Geometry: see drawing. Coordinates: mm, zero at the bounding-box minimum. A direction names the side the tool comes from. Give positions to 0.01 mm unless a question says otherwise; leave off trailing zeros. Write each loop counter-clockwise with the first axis right and the second up, starting at its lowest first coordinate (ties: lowest second). Pieces come first, ordered by that corner, then holes. Notation, with made-up numbers: M 64,38 L 95,38 A28 cw 95,67 Z; hole C 31,-34 d7. An arc over 180 degrees is marked long. Answer as a JSON object with one key per item and string values. Group by question number.
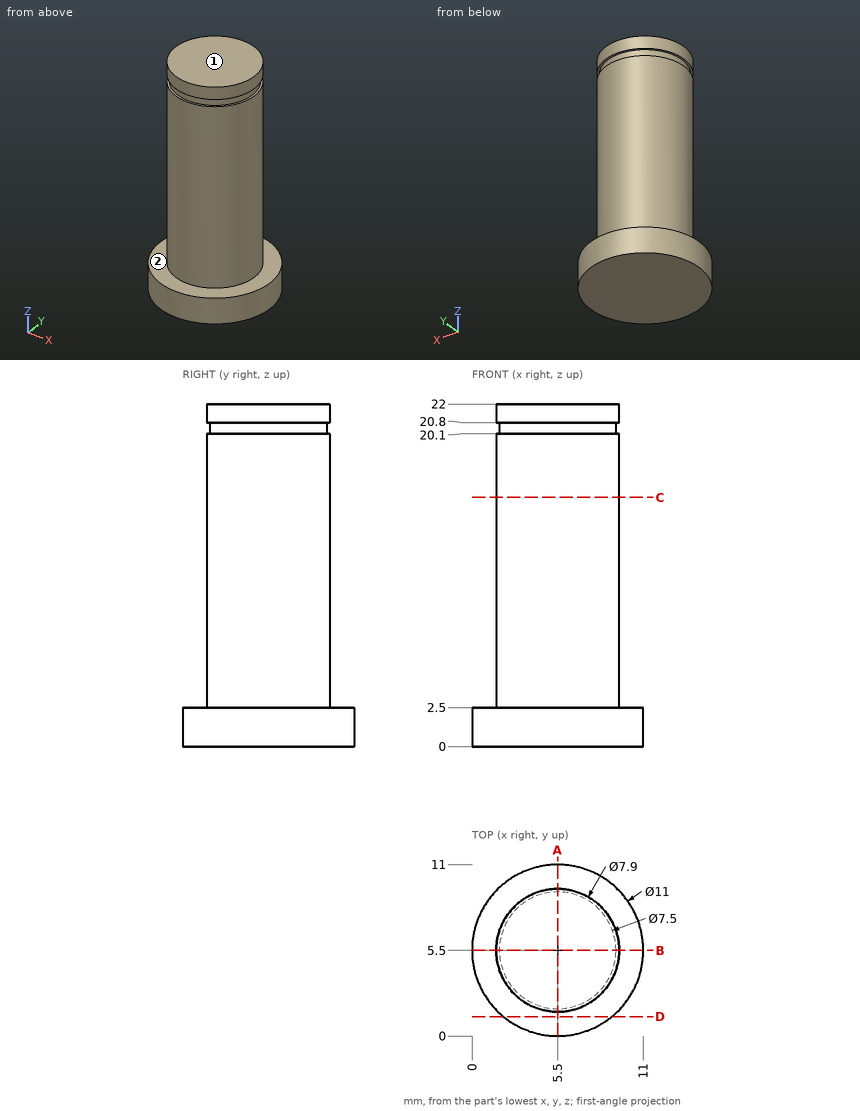
(1) Access query for the marked faces 1 and 2. Directions: +Z, -Z, +X, -X, +Y, -Y. A direction counts if a zero-diameter tool reaches every point of the face in a straight line with its end or side. Return the directions, or none.
(2) Section C-C, the plane z = 16. Return loops of the section in (x, y).
(3) Section D-D, the plane y = 1.25. Return loops of the section in (x, z), plus the area to 3 significant figures.
(4) Ray query, L1, parallel to Z at x = 8.5, y = 8; L2, parallel to Z at x = 7.75, y = 9; L3, parallel to Y at x = 6.75, z = 16.25. Return the intervals inside material, ascending. Write a range as [from, to].
(5) Contact query for flat-ended pins moving along their axis: pin 1 Ø2 at (y, z) = (3.5, 3) entering from -X; pin 2 Ø4 at (y, z) = (1.5, 15) entering from +X; pin 3 Ø2 at (y, z) = (6, 6.5) entering from -X. Output: stop coordinate, or through.
(6) Section A-A, the plane x = 5.5. Return loops of the section in (y, z).
Reported:
{
 "1": {"face 1": "+Z, +X, -X, +Y, -Y", "face 2": "+Z"},
 "2": {"outline": "C 5.5,5.5 d7.9"},
 "3": {"outline": "M 2.01,0 L 8.99,0 L 8.99,2.5 L 2.01,2.5 Z", "area": "17.5 mm2"},
 "4": {"L1": "z = [0, 20.1], [20.8, 22]", "L2": "z = [0, 2.5]", "L3": "y = [1.75, 9.25]"},
 "5": {"pin 1": "stops at x = 0.12", "pin 2": "stops at x = 8.91", "pin 3": "stops at x = 1.55"},
 "6": {"outline": "M 0,0 L 11,0 L 11,2.5 L 9.45,2.5 L 9.45,20.1 L 9.25,20.1 L 9.25,20.8 L 9.45,20.8 L 9.45,22 L 1.55,22 L 1.55,20.8 L 1.75,20.8 L 1.75,20.1 L 1.55,20.1 L 1.55,2.5 L 0,2.5 Z"}
}
